Autodesk Inventor part; units mm, degrees
ref_plane "YZ Plane" through (0, 0, 0) normal (1, 0, 0) x (0, 1, 0)
ref_plane "XZ Plane" through (0, 0, 0) normal (0, 1, 0) x (-1, 0, 0)
ref_plane "XY Plane" through (0, 0, 0) normal (0, 0, 1) x (1, 0, 0)
sketch "スケッチ1" plane through (0, 0, 0) normal (0, 0, 1) x (1, 0, 0)
  line L0 (0, 0) -> (15, 0)
  line L1 (15, 0) -> (15, 15)
  line L2 (15, 15) -> (0, 15)
  line L3 (0, 15) -> (0, 0)
  dimension "d0" = 15
  dimension "d1" = 15
extrude "押し出し1" add sketch "スケッチ1" along normal blind 825
sketch "スケッチ2" plane through (0, 15, 825) normal (0, 1, 0) x (1, 0, 0)
  line L0 (15, 0) -> (0, 0)
  line L1 (15, 825) -> (15, 0)
  point P0 (0, 825)
  point P1 (7.5, 310)
  point P2 (7.5, 320)
  point P3 (7.5, 330)
  point P4 (7.5, 432.5)
  point P5 (7.5, 442.5)
  point P6 (7.5, 452.5)
  point P7 (7.5, 495)
  point P8 (7.5, 505)
  point P9 (7.5, 515)
  point P10 (7.5, 610)
  point P11 (7.5, 620)
  point P12 (7.5, 630)
  point P13 (7.5, 732.5)
  point P14 (7.5, 742.5)
  point P15 (7.5, 752.5)
  point P16 (7.5, 795)
  point P17 (7.5, 805)
  point P18 (7.5, 815)
  point P19 (7.5, 215)
  point P20 (7.5, 205)
  point P21 (7.5, 195)
  point P22 (7.5, 152.5)
  point P23 (7.5, 142.5)
  point P24 (7.5, 132.5)
  point P25 (7.5, 30)
  point P26 (7.5, 20)
  point P27 (7.5, 10)
  dimension "d4" = 310
  dimension "d5" = 7.5
  dimension "d6" = 10
  dimension "d7" = 10
  dimension "d8" = 102.5
  dimension "d9" = 10
  dimension "d10" = 10
  dimension "d11" = 42.5
  dimension "d12" = 10
  dimension "d13" = 10
  dimension "d14" = 95
  dimension "d15" = 10
  dimension "d16" = 10
  dimension "d17" = 102.5
  dimension "d18" = 10
  dimension "d19" = 10
  dimension "d20" = 42.5
  dimension "d21" = 10
  dimension "d22" = 10
  dimension "d23" = 95
  dimension "d24" = 10
  dimension "d25" = 10
  dimension "d26" = 42.5
  dimension "d27" = 10
  dimension "d28" = 10
  dimension "d29" = 102.5
  dimension "d30" = 10
  dimension "d31" = 10
hole "穴1" at (7.5, 15, 515) at (7.5, 15, 505) at (7.5, 15, 495) at (7.5, 15, 392.5) at (7.5, 15, 382.5) at (7.5, 15, 372.5) at (7.5, 15, 330) at (7.5, 15, 320) at (7.5, 15, 310) at (7.5, 15, 215) at (7.5, 15, 205) at (7.5, 15, 195) at (7.5, 15, 92.5) at (7.5, 15, 82.5) at (7.5, 15, 72.5) at (7.5, 15, 30) at (7.5, 15, 20) at (7.5, 15, 10) at (7.5, 15, 610) at (7.5, 15, 620) at (7.5, 15, 630) at (7.5, 15, 672.5) at (7.5, 15, 682.5) at (7.5, 15, 692.5) at (7.5, 15, 795) at (7.5, 15, 805) at (7.5, 15, 815) direction (0, -1, 0) diameter 3.2 end through all
Check sheet for the modelled part. Datum: model origin and axes. Units: mm. Round coordinates to 2 decimals unless told otherwise and drop trailing zeros.
1) Section check A-A (y = 10.5). Give the number of separate pieces and of enclosed holes in the cut face, and give its area (3 significant figures).
2) Go/stop test with a flat-tipped pin: pin 1 Ø1.9 at (x, z) = (7.5, 505) entering from -Y. Record where the tip stops, or that it passes through.
3) Scan line: line 1 (X direction, y = 8.5, z = 10). Record every from-to range of solid material in increasing order.
Result:
1. separate pieces: 1
1. enclosed holes: 27
1. area: 12,200 mm2
2. pin 1: passes through
3. line 1: x = 0 to 5.9, 9.1 to 15
